Source: CAD feature listing. Evaluate the final solid. Frame: model axes, mm. Give positions to 0.01 mm unless a question says otherwise; leave off trailing zeros. Write each loop counter-clockwise with the first axis right and the second up, starting at its lowest first coordinate (ties: lowest second). Pieces come first, ordered by that corner, then holes. Notation, with made-up numbers: (60, 24.25) - (113, 24.25) arc R27 cw to (113, 59.25) - close; hole circle Ø6 at (24.5, 51.25). An arc over 180 degrees is marked (long way). Answer as a JSON object with one key per item and string values. Group by question number.
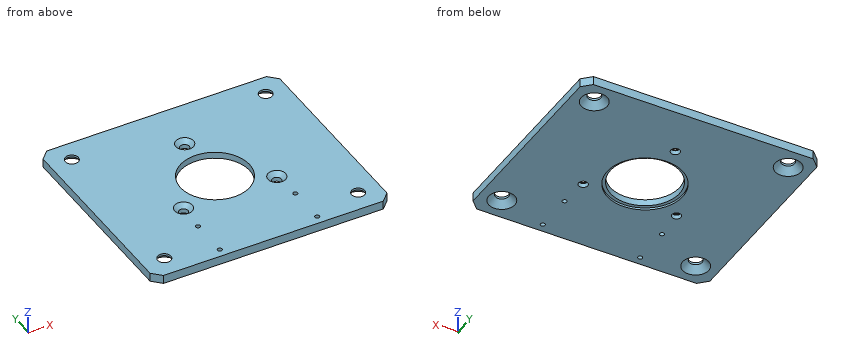
from build123d import *

# Parameters (mm, degrees)
SKETCH_1_W               = 110
SKETCH_1_H               = 96.2
SKETCH_1_R               = 3.05
SKETCH_1_R_2             = 16
EXTRUDE_1_DEPTH          = 2
CHAMFER_1_SIZE           = 4
CHAMFER_2_SIZE           = 3
SKETCH_2_R               = 17.5
CUT_EXTRUDE_1_DEPTH      = 1
SKETCH_3_R               = 2.1
CUT_EXTRUDE_2_DEPTH      = 74.175200717
PATTERN_CIRCULAR_1_COUNT = 3
CHAMFER_3_SIZE           = 2
SKETCH_4_R               = 1.05
CUT_EXTRUDE_3_DEPTH      = 74.175200717


with BuildPart() as part:
    # 草图1 → 凸台-拉伸1 (new, symmetric)
    with BuildSketch(Plane.XY):
        Rectangle(SKETCH_1_W, SKETCH_1_H)
        with Locations((-45, 38.1)):
            Circle(SKETCH_1_R, mode=Mode.SUBTRACT)
        with Locations((-45, -38.1)):
            Circle(SKETCH_1_R, mode=Mode.SUBTRACT)
        with Locations((45, -38.1)):
            Circle(SKETCH_1_R, mode=Mode.SUBTRACT)
        with Locations((45, 38.1)):
            Circle(SKETCH_1_R, mode=Mode.SUBTRACT)
        Circle(SKETCH_1_R_2, mode=Mode.SUBTRACT)
    extrude(amount=EXTRUDE_1_DEPTH, both=True)

    # 倒角1
    chamfer_1_edges = [part.edges().sort_by_distance(p)[0] for p in [
        (-55, 48.1, 0),
        (55, 48.1, 0),
        (55, -48.1, 0),
        (-55, -48.1, 0),
    ]]
    chamfer(chamfer_1_edges, length=CHAMFER_1_SIZE)

    # 倒角2
    chamfer_2_edges = [part.edges().sort_by_distance(p)[0] for p in [
        (-48.05, 38.1, -2),
        (-48.05, -38.1, -2),
        (41.95, -38.1, -2),
        (41.95, 38.1, -2),
    ]]
    chamfer(chamfer_2_edges, length=CHAMFER_2_SIZE)

    # 草图2 → 切除-拉伸1 (cut)
    with BuildSketch(Plane(origin=(0, 0, -2), x_dir=(-1, 0, 0), z_dir=(0, 0, -1))):
        Circle(SKETCH_2_R)
    extrude(amount=-CUT_EXTRUDE_1_DEPTH, mode=Mode.SUBTRACT)

    # 草图3 → 切除-拉伸2 (cut, through all)
    with BuildSketch(Plane(origin=(0, 0, -2), x_dir=(-1, 0, 0), z_dir=(0, 0, -1))):
        with Locations((0, 25)):
            Circle(SKETCH_3_R)
    cut_extrude_2 = extrude(amount=-CUT_EXTRUDE_2_DEPTH, mode=Mode.SUBTRACT)

    # 阵列(圆周)1: 切除-拉伸2 ×3 about axis
    pattern_circular_1_axis = Axis((0, 0, 0), (0, 0, 1))
    for i in range(1, PATTERN_CIRCULAR_1_COUNT):
        add(cut_extrude_2.rotate(pattern_circular_1_axis, i * 360 / PATTERN_CIRCULAR_1_COUNT), mode=Mode.SUBTRACT)

    # 倒角3
    chamfer_3_edges = [part.edges().sort_by_distance(p)[0] for p in [
        (2.1, 25, 2),
        (-22.700635095, -10.681346652, 2),
        (20.600635095, -14.318653348, 2),
    ]]
    chamfer(chamfer_3_edges, length=CHAMFER_3_SIZE)

    # 草图4 → 切除-拉伸3 (cut, through all)
    with BuildSketch(Plane(origin=(0, 0, -2), x_dir=(-1, 0, 0), z_dir=(0, 0, -1))):
        with Locations((-22.6, -26.1)):
            Circle(SKETCH_4_R)
        with Locations((-22.6, -44.1)):
            Circle(SKETCH_4_R)
        with Locations((22.6, -26.1)):
            Circle(SKETCH_4_R)
        with Locations((22.6, -44.1)):
            Circle(SKETCH_4_R)
    extrude(amount=-CUT_EXTRUDE_3_DEPTH, mode=Mode.SUBTRACT)


solid = part.part
Q1. Section B-B on y = -38.1. Return the cut outline in (x, z), then the cut area to 3 significant figures.
Q2. Ray query, probe 1 along Y at (x, z) = (-45, 1.2); probe 2 along Y at (x, z) = (0, -1.2); probe 3 along X at (y, z) = (35, -0.4). Return the intervals inside material, ascending. Write a range as [from, to].
Q3. First-contact query: pin 1 Ø2.5 at (x, y) = (-22.6, -44.1) entering from +Z; pin 2 Ø10.5 at (x, y) = (7, 4) entering from -Z; pin 3 Ø10 at (x, y) = (45, 38.1) entering from -Z; pin 4 Ø5.5 at (x, y) = (0, 25) entering from +Z. Flat tips, straight axial feed; report the tip coordinate or a pass-through.
Q4. Section A-A on x = 0. Return the cut outline in (y, z).
Q5. Section D-D on y = 25. Return the cut outline in (x, z).
Q6. Section C-C on y = 0. Return the cut outline in (x, z).
Taken from the geometry:
{
 "1": {"outline": "(-55, -2) - (-51.05, -2) - (-48.05, 1) - (-48.05, 2) - (-55, 2) - close; (-41.95, 1) - (-38.95, -2) - (38.95, -2) - (41.95, 1) - (41.95, 2) - (-41.95, 2) - close; (48.05, 1) - (51.05, -2) - (55, -2) - (55, 2) - (48.05, 2) - close", "area": "373 mm²"},
 "2": {"probe 1": "y = [-48.1, -41.15], [-35.05, 35.05], [41.15, 48.1]", "probe 2": "y = [-48.1, -17.5], [17.5, 22.9], [27.1, 48.1]", "probe 3": "x = [-55, -48.19], [-41.81, 41.81], [48.19, 55]"},
 "3": {"pin 1": "stops at z = 2", "pin 2": "passes through", "pin 3": "stops at z = -0.95", "pin 4": "stops at z = 0.65"},
 "4": {"outline": "(-48.1, -2) - (-17.5, -2) - (-17.5, -1) - (-16, -1) - (-16, 2) - (-48.1, 2) - close; (16, -1) - (17.5, -1) - (17.5, -2) - (22.9, -2) - (22.9, 0) - (20.9, 2) - (16, 2) - close; (27.1, -2) - (48.1, -2) - (48.1, 2) - (29.1, 2) - (27.1, 0) - close"},
 "5": {"outline": "(-55, -2) - (-2.1, -2) - (-2.1, 0) - (-4.1, 2) - (-55, 2) - close; (2.1, -2) - (55, -2) - (55, 2) - (4.1, 2) - (2.1, 0) - close"},
 "6": {"outline": "(-55, -2) - (-17.5, -2) - (-17.5, -1) - (-16, -1) - (-16, 2) - (-55, 2) - close; (16, -1) - (17.5, -1) - (17.5, -2) - (55, -2) - (55, 2) - (16, 2) - close"}
}
